Answer from the drawing. Dimensions are ordinates in mm from the lowest x, y and z of the part. A direction names the side the tool comes from. Coordinates: 2 decimals unless noted, no trailing zeros. Write each loop counter-clockwise with the first axis right and the second up, starting at its lowest first coordinate (ties: lowest second). Pieces come first, ordered by that corner, then holes. Notation, with made-up numbers: (40, 61) -> (59, 61) arc R6 ccw to (59, 72) -> close; hole circle Ø9 at (17.25, -6). An arc over 180 degrees is marked (long way). Return JSON: item names as keys, results as strings.
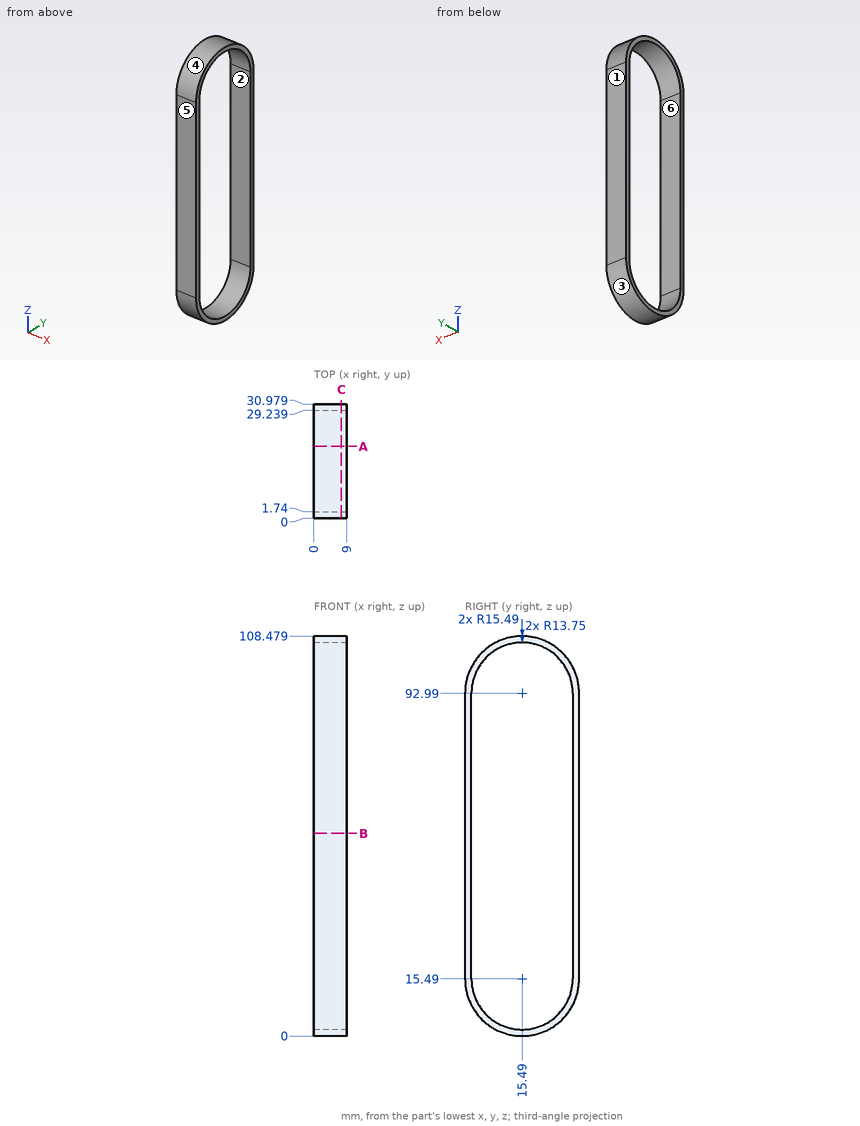
1. The part is cut by section A-A (y = 19.5). Determine the outline of the cut face in (x, z).
Taken from the geometry:
{"outline": "(0, 0.53) -> (9, 0.53) -> (9, 2.34) -> (0, 2.34) -> close; (0, 106.14) -> (9, 106.14) -> (9, 107.95) -> (0, 107.95) -> close"}
2. For a pull along Z with two mould halves and no side action, classify the marked faces 1, 2, 3 and 4 as +Z half, -Z half, draft (parallel to the pull), parting line (faces both ways), or undercut.
Taken from the geometry:
{"face 1": "draft", "face 2": "undercut", "face 3": "-Z half", "face 4": "+Z half"}
3. The part is cut by section B-B (z = 55). Determine the outline of the cut face in (x, y).
Taken from the geometry:
{"outline": "(0, 0) -> (9, 0) -> (9, 1.74) -> (0, 1.74) -> close; (0, 29.24) -> (9, 29.24) -> (9, 30.98) -> (0, 30.98) -> close"}
4. The part is cut by section C-C (x = 7.5). Determine the outline of the cut face in (y, z).
Taken from the geometry:
{"outline": "(0, 15.49) arc R15.49 ccw to (30.98, 15.49) -> (30.98, 92.99) arc R15.49 ccw to (0, 92.99) -> close; hole (1.74, 15.49) arc R13.75 ccw to (29.24, 15.49) -> (29.24, 92.99) arc R13.75 ccw to (1.74, 92.99) -> close"}
5. Consider L1, parallel to Y at x = 6.25, z = 29; L2, parallel to Z at x = 6.25, y = 16; L3, parallel to Z at x = 5.5, y = 10.5 (1 decimal). Determine where each line is inside the solid, lowest interval first.
Taken from the geometry:
{"L1": "y = 0 to 1.74, 29.24 to 30.98", "L2": "z = 0.01 to 1.75, 106.73 to 108.47", "L3": "z = 0.8 to 2.7, 105.8 to 107.7"}
6. A tool of negligible diameter and unlimited length cuts with its end or side. For the marked faces 5 and 6, from which of +Z, -Z, +X, -X, +Y, -Y can it reach the whole face along a straight path? Write none if from no direction.
Taken from the geometry:
{"face 5": "+Z, -Z, +X, -X, -Y", "face 6": "+X, -X"}
